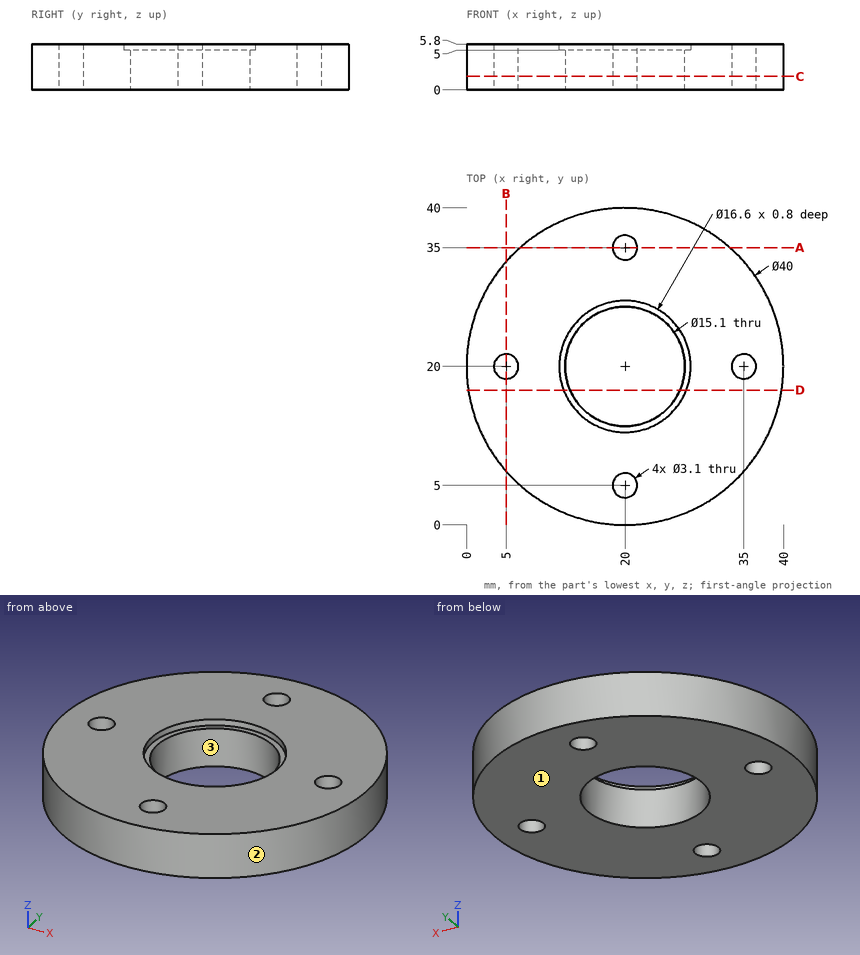
Here's the drawing with two shaded views (mm, measured from the low corner). I have some questions. Give positions to 0.01 mm unless a question says otherwise; leave off trailing zeros. Order: outer loops, then holes, each group sorted by start corner. A loop starts at its lowest first (then second) coordinate and runs counter-clockwise, first axis right, second up. Notation, with made-up numbers: M 83,20 L 106,20 A21 cw 106,32 Z; hole C 14.25,-6 d5. An arc over 180 degrees is marked long. One line per item, written item: value.
1) We'd pull the mould along X, two halves only. Please class the marked faces 1, 2 and 3: released by +X, released by -X, zero draft, split by the parting line, or undercut.
Answer sheet:
face 1: zero draft
face 2: split by the parting line
face 3: undercut
2) For P1, Ø2, axis at y = 7.5, z = 4, coming from the -X side, with a flat end and sliding along its axis, tell me the tip position at first contact or that it passes through.
Answer sheet:
P1: stops at x = 3.64
3) I want a section at A-A, the plane y = 35. List the corners of the cut face in (x, z) for me.
Answer sheet:
outline: M 6.77,0 L 18.45,0 L 18.45,5.8 L 6.77,5.8 Z; M 21.55,0 L 33.23,0 L 33.23,5.8 L 21.55,5.8 Z
4) I want a section at C-C, the plane z = 1.7. List the corners of the cut face in (x, y) for me.
Answer sheet:
outline: C 20,20 d40; hole C 5,20 d3.1; hole C 20,20 d15.1; hole C 20,5 d3.1; hole C 20,35 d3.1; hole C 35,20 d3.1
5) I want a section at D-D, the plane y = 17. List the corners of the cut face in (x, z) for me.
Answer sheet:
outline: M 0.23,0 L 13.07,0 L 13.07,5 L 12.26,5 L 12.26,5.8 L 0.23,5.8 Z; M 26.93,0 L 39.77,0 L 39.77,5.8 L 27.74,5.8 L 27.74,5 L 26.93,5 Z
6) Please list where these lines run through material, in increasing order: line 1 along Y through (x, z) = (20, 4.15); line 2 along Y through (x, z) = (20, 5.35); line 3 along Y through (x, z) = (18, 2.1).
Answer sheet:
line 1: y = 0 to 3.45, 6.55 to 12.45, 27.55 to 33.45, 36.55 to 40
line 2: y = 0 to 3.45, 6.55 to 11.7, 28.3 to 33.45, 36.55 to 40
line 3: y = 0.1 to 12.72, 27.28 to 39.9
